Part model, mm, in its own coordinate system. Face numbers are marked on the shaded views. Give positions to 0.01 mm unless a question says otherwise; leave off trailing zeros. Write each loop counter-clockwise with the first axis right and the second up, starting at its lowest first coordinate (ties: lowest second). Pieces come first, ordered by that corner, then holes. Notation, with made-up numbers: M 29.25,65.5 L 70.25,65.5 A8 cw 70.25,70.5 Z; hole C 5.5,5 d6. An arc over 180 degrees is marked long. Use a Markdown table: item, result.
Autodesk Inventor part; units mm, degrees
ref_plane "YZ Plane" through (0, 0, 0) normal (1, 0, 0) x (0, 1, 0)
ref_plane "XZ Plane" through (0, 0, 0) normal (0, 1, 0) x (-1, 0, 0)
ref_plane "XY Plane" through (0, 0, 0) normal (0, 0, 1) x (1, 0, 0)
sketch "Sketch1" plane through (0, 0, 0) normal (0, 0, 1) x (1, 0, 0)
  line L0 (0, 25.4) -> (-28.702, 25.4) construction
  line L1 (0, 25.4) -> (-95.25, 25.4) construction
  line L2 (-95.25, 25.4) -> (-92.075, 25.4) construction
  line L3 (-92.075, 25.4) -> (-84.455, 21.8467) construction
  line L4 (-92.075, 25.4) -> (-92.075, 22.4389) construction
  line L5 (-92.075, 0) -> (-95.25, 0)
  line L6 (-28.702, 59.0535) -> (-28.702, -92.5226) construction
  arc A0 (-28.9184, -9.8402) -> (-32.3684, -2.4417) centre (-35.052, -8.1967) ccw
  line L7 (-76.2, -186.2977) -> (-28.702, -9.0327)
  line L8 (-92.075, 25.4) -> (-92.075, 0)
  line L9 (-92.075, 25.4) -> (-32.3684, -2.4417)
  line L10 (-28.702, -8.1967) -> (-60.452, -8.1967) construction
  line L11 (-60.452, -127.5253) -> (-54.102, -127.5253) construction
  line L12 (-54.102, -127.5253) -> (-54.102, -103.8268) construction
  line L13 (-54.102, -103.8268) -> (-60.452, -103.8268)
  line L14 (-60.452, 10.654) -> (-60.452, 1.129) construction
  line L15 (-60.452, 10.654) -> (-60.452, 4.1232) construction
  line L16 (-60.452, 4.1232) -> (-46.4468, 4.1232)
  line L17 (-95.25, 0) -> (-95.25, -12.7) construction
  line L18 (-60.452, -12.7) -> (-73.152, -12.7) construction
  line L19 (-95.25, -12.7) -> (-95.25, -25.4) construction
  line L20 (-95.25, -25.4) -> (-95.25, -88.9) construction
  line L21 (-95.25, -88.9) -> (-82.55, -88.9) construction
  line L22 (-82.55, -88.9) -> (-82.55, -25.4) construction
  line L23 (-95.25, -25.4) -> (-82.55, -25.4)
  line L24 (-82.55, -25.4) -> (-82.55, -88.9)
  line L25 (-82.55, -88.9) -> (-95.25, -88.9)
  line L26 (-95.25, -12.7) -> (-73.152, -12.7)
  line L27 (-73.152, -139.3746) -> (-63.627, -139.3746)
  line L28 (-82.55, -88.9) -> (-82.55, -186.2977)
  line L29 (-82.55, -186.2977) -> (-76.2, -186.2977)
  line L30 (-73.152, -12.7) -> (-73.152, -139.3746)
  line L31 (-88.9, -25.4) -> (-88.9, -31.3436)
  line L32 (-88.9, -31.3436) -> (-95.25, -31.3436)
  line L33 (-95.25, 0) -> (-95.25, -25.4)
  line L34 (-95.25, -31.3436) -> (-95.25, -88.9)
  line L35 (-88.9, -160.8977) -> (-88.9, -221.8454)
  line L36 (-28.9184, -9.8402) -> (-85.725, -221.8454)
  line L37 (-85.725, -221.8454) -> (-88.9, -221.8454)
  line L38 (-82.55, -160.8977) -> (-88.9, -160.8977)
  line L39 (-66.802, -38.1) -> (-66.802, 4.1232)
  line L40 (-66.802, 4.1232) -> (-60.452, 4.1232)
  line L41 (-66.802, -38.1) -> (-60.452, -103.8268)
  line L42 (-60.452, 10.654) -> (-60.452, 4.1232) construction
  line L43 (-60.452, -8.1967) -> (-60.452, -12.7) construction
  line L44 (-60.452, -103.8268) -> (-60.452, -127.5253) construction
  line L45 (0, 59.6457) -> (0, -91.9304) construction
  line L46 (-73.152, -38.1) -> (-69.977, -38.1)
  line L47 (-69.977, -38.1) -> (-69.977, -12.7)
  line L48 (-66.802, -12.7) -> (-69.977, -12.7)
  point P0 (0, 0)
  point P1 (-95.25, -256.5049)
  point P2 (-88.7095, 22.4389)
  dimension "d0" = 28.702
  dimension "d1" = 95.25
  dimension "d2" = 3.175
  dimension "d3" = 25
  dimension "d5" = 25.4
  dimension "d6" = 25.4
  dimension "d8" = 12.7
  dimension "d12" = 31.75
  dimension "d13" = 6.35
  dimension "d16" = 12.7
  dimension "d17" = 12.7
  dimension "d18" = 12.7
  dimension "d19" = 63.5
  dimension "d20" = 12.7
  dimension "d22" = 9.525
  dimension "d23" = 6.35
  dimension "d25" = 5.9436
  dimension "d27" = 3.175
  dimension "d28" = 6.35
  dimension "d29" = 25.4
  dimension "d30" = 107.95
  dimension "d31" = 6.35
  dimension "d33" = 20.3552
  dimension "d34" = 15
  dimension "d35" = 3.175
  dimension "d36" = 25.4
revolve "Revolution1" add sketch "Sketch1" angle 360 about axis through (0, 59.6457, 0) along (0, -1, 0) contours L26 L30 L27 L7 L29 L28 L24 L23 L33
properties part number "aluminum_casing" material "Aluminum 6061"
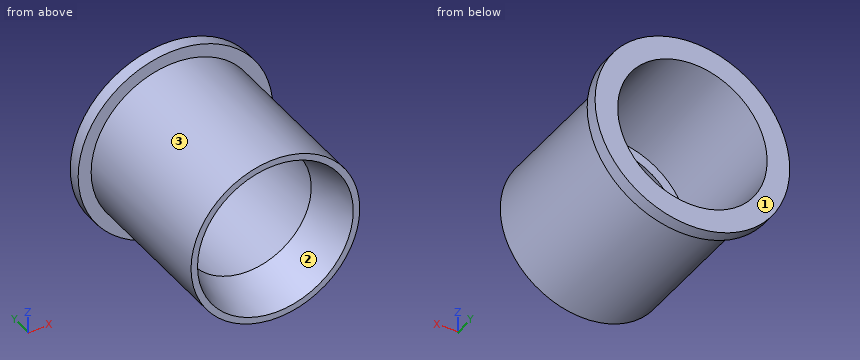
1. Drop flat-ended pins along their axis: P1, Ø1, axis at y = -120, z = -41, coming from the -X side; P2, Ø12, axis at x = 1, z = 61.5, coming from the +Y side; P3, Ø1, axis at x = -5, y = -167.5, coming from the -Z side. Give the stop position or say it passes through.
Findings below:
| item | result |
|---|---|
| P1 | x = -71.93 |
| P2 | y = -139.37 |
| P3 | z = -82.43 |
2. Two-plate mould, pull along Z, no slides. Class the marked faces 1, 2 and 3: released by +Z, released by -Z, zero draft, split by the parting line, or undercut.
Findings below:
| item | result |
|---|---|
| face 1 | zero draft |
| face 2 | undercut |
| face 3 | split by the parting line |
3. Cut at D-D, the plane y = -65. Give the cut face in (x, z), then the cut area to 3 significant figures.
Findings below:
| item | result |
|---|---|
| outline | C 0,0 d165.1; hole C 0,0 d146.3 |
| area | 4,600 mm2 |
4. Drill centre lines: L1, parallel to Z at x = 0, y = -60; L2, parallel to Y at x = 53.5, z = 74. Where is each one in solid material? Low to high.
Findings below:
| item | result |
|---|---|
| L1 | -82.55 to -73.15, 73.15 to 82.55 |
| L2 | -25.4 to -12.7 |
5. Cut at B-B, the plane z = 0. Give the cut face in (x, y).
Findings below:
| item | result |
|---|---|
| outline | M -95.25,-25.4 L -82.55,-25.4 L -82.55,-186.3 L -76.2,-186.3 L -63.63,-139.37 L -73.15,-139.37 L -73.15,-12.7 L -95.25,-12.7 Z; M 63.63,-139.37 L 76.2,-186.3 L 82.55,-186.3 L 82.55,-25.4 L 95.25,-25.4 L 95.25,-12.7 L 73.15,-12.7 L 73.15,-139.37 Z |
6. Cut at C-C, the plane y = -149.5. Give the cut face in (x, z).
Findings below:
| item | result |
|---|---|
| outline | C 0,0 d165.1; hole C 0,0 d132.68 |
7. Cut at A-A, the plane x = 0. Give the cut face in (y, z).
Findings below:
| item | result |
|---|---|
| outline | M -186.3,-82.55 L -25.4,-82.55 L -25.4,-95.25 L -12.7,-95.25 L -12.7,-73.15 L -139.37,-73.15 L -139.37,-63.63 L -186.3,-76.2 Z; M -186.3,76.2 L -139.37,63.63 L -139.37,73.15 L -12.7,73.15 L -12.7,95.25 L -25.4,95.25 L -25.4,82.55 L -186.3,82.55 Z |
